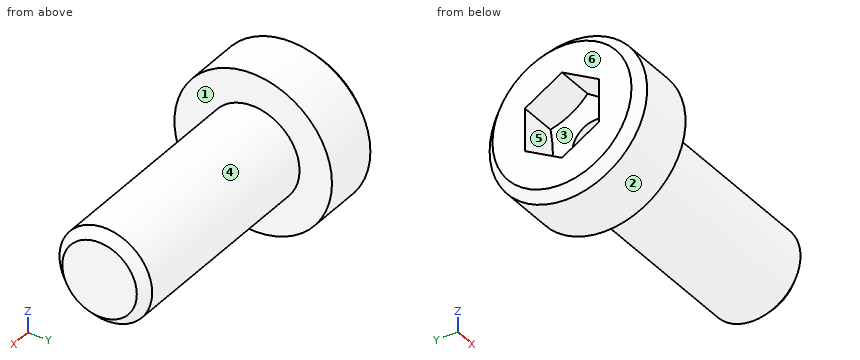
Autodesk Inventor part; units mm, degrees
ref_plane "Work Plane1" through (6, 0, 0) normal (0, 0.5, 0.8660254) x (1, 0, 0)
ref_plane "YZ Plane" through (0, 0, 0) normal (1, 0, 0) x (0, 1, 0)
ref_plane "XZ Plane" through (0, 0, 0) normal (0, 1, 0) x (-1, 0, 0)
sketch "Sketch1" plane through (0, 0, 0) normal (0, 0, 1) x (1, 0, 0)
  line L0 (1.2217, 0) -> (12, 0)
  line L1 (12, 0) -> (12, 2.5)
  line L2 (12, 2.5) -> (0, 2.5)
  line L3 (0, 2.5) -> (0, 4.25)
  line L4 (0, 4.25) -> (-3.5, 4.25)
  line L5 (-3.5, 4.25) -> (-3.5, 2.3094)
  line L6 (-3.5, 2.3094) -> (-1.5, 2.3094)
  line L7 (-1.5, 2.3094) -> (-0.8884, 1.25)
  line L8 (-6.6, 0) -> (15.1, 0)
  line L9 (0, -0.85) -> (0, 5.1)
  line L10 (-0.8884, 1.25) -> (0.5, 1.25)
  line L11 (0.5, 1.25) -> (1.2217, 0)
  line L12 (-3.5, 2.3094) -> (-3.5, 0) construction
  line L13 (-3.5, 3.75) -> (-3, 4.25)
  dimension "d0" = 3.5
  dimension "d1" = 2
  dimension "d2" = 60
  dimension "d3" = 5
  dimension "d4" = 4.6188
  dimension "d5" = 8.5
  dimension "d15" = 4
  dimension "d16" = 2.5
  dimension "d17" = 12
  dimension "d32" = 45
  dimension "d33" = 0.5
revolve "Body" add sketch "Sketch1" angle 360 about axis through (1.2217, 0, 0) along (1, 0, 0) contours L11 L10 L9 L2 L1 L0 | L10 L7 L6 L5 L13 L4 L3 L9 | L13 L5 L4
revolve "Chamfer2" cut sketch "Sketch1" angle 360 about axis through (-10, 0, 0) along (1, 0, 0) contours L13 L5 L4
sketch "Sketch2" plane through (-3.5, 0, 0) normal (-1, 0, 0) x (0, 0, 1)
  circle A0 centre (0, 0) radius 2.3094
  line L0 (0, -5.95) -> (0, 5.95)
  line L1 (-5.95, 0) -> (5.95, 0)
  line L2 (2.3094, 0) -> (1.1547, -2)
  line L3 (1.1547, -2) -> (-1.1547, -2)
  line L4 (-1.1547, -2) -> (-2.3094, 0)
  line L5 (-2.3094, 0) -> (-1.1547, 2)
  line L6 (-1.1547, 2) -> (1.1547, 2)
  line L7 (1.1547, 2) -> (2.3094, 0)
extrude "Slot" add sketch "Sketch2" against normal up to next contours L7 A0 | A0 L2 | L6 L0 A0 | A0 L0 L3 | L0 L6 A0 | A0 L3 L0 | L4 A0 | A0 L5
thread "Thread"
chamfer "Chamfer1" distance 0.4908 distance2 0.4908 1 edges at (12, -2.5, 0) measured on face at (12, -0.7741, -0.6858)
ref_plane "Work Plane1" through (6, 0, 0) normal (0, 0.5, 0.8660254) x (1, 0, 0)
equation "\"d0\" = KOH"
equation "\"d1\" = INTI"
equation "\"d3\" = GD"
equation "\"d4\" = 1.1547 * SW"
equation "\"d5\" = KOD"
equation "\"d15\" = INFT"
equation "\"d16\" = SDT"
equation "\"d17\" = NLG"
equation "\"d33\" = Cham"
equation "\"d7\" = GEL"
equation "\"d9\" = -0.5 * SPD + 0.5 * GD"
equation "\"d12\" = GUL"
equation "\"GD\" = NND"
equation "\"NLG\" = 12"
equation "\"GEL\" = 7.8"
equation "\"KOD\" = 8.5"
equation "\"KOH\" = 3.5"
equation "\"GUL\" = 0.61345 * PTC"
equation "\"SW\" = 4"
equation "\"INTI\" = 2"
equation "\"SPD\" = NND - 1.2269 * PTC"
equation "\"SDT\" = 2.5"
equation "\"INFT\" = 4"
equation "\"Cham\" = 0.5"
equation "\"TOA\" = 30deg"
equation "\"GD1\" = THREADDIA - 1.2269 * PTC"
equation "\"THREADDIA\" = 5"
equation "\"BDM\" = NND"
equation "\"FAWI\" = 45deg"
equation "\"RR\" = 0.1 * NND"
equation "\"PTC\" = 0.8"
equation "\"NND\" = 5"
equation "\"FAWI1\" = 45deg"
equation "\"GAL\" = 0.61345 * PTC"
equation "\"E0\" = 1.155 * SW"
properties part number "DIN 6912 - M5 x 12" material "Steel, Mild"
Geometry: final body of the model. Coordinates: model frame, mm. Face numbers are marked on the shaded views. A direction names the side the tool comes from. Give positions to 0.01 mm unless a question says otherwise; leave off trailing zeros. Write each loop counter-clockwise with the first axis right and the second up, starting at its lowest first coordinate (ties: lowest second). Pieces come first, ordered by that corner, then holes. Notation, with made-up numbers: (27, 86) - (53, 86) arc R23 cw to (53, 103) - close; hole circle Ø8 at (54.25, 30.5). An arc over 180 degrees is marked (long way). Return JSON: item names as keys, results as strings. Group by question number.
1) Mould query, pull axis Z, two halves, no side actions, for the marked faces 1, 2 and 3. Classes: released by +Z, released by -Z, zero draft, split by the parting line, or undercut.
2) Set-up query: the marked faces 4, 5 and 6. Return all of +Z, -Z, +X, -X, +Y, -Y with unobstructed straight access to the full face (end or side cutting, diameter ignored); none if empty.
3) Line query: line 1 (Z direction, x = 0.15, y = 0); line 2 (Z direction, x = -0.55, y = 0); line 3 (X direction, y = -2.5, z = 1.5). Output: solid intervals per line, ascending.
4) Section B-B on x = 6.25. Return the cut outline in (y, z).
5) First-contact query: P1, Ø1.5, axis at y = 2, z = 1.5, coming from the +X side; P2, Ø1, axis at x = 4, z = 0, coming from the -Y side; P3, Ø1.5, axis at y = 0, z = 0, coming from the -X side. Flat tips, straight axial feed; report the tip coordinate or a pass-through.
6) Section A-A on x = 0.25. Return the cut outline in (y, z), plus the area to 3 significant figures.
Filled in:
{
 "1": {"face 1": "zero draft", "face 2": "split by the parting line", "face 3": "undercut"},
 "2": {"face 4": "+X", "face 5": "-X", "face 6": "+Z, -Z, -X, +Y, -Y"},
 "3": {"line 1": "z = -2.5 to -1.25, 1.25 to 2.5", "line 2": "z = -4.25 to -1.25, 1.25 to 4.25", "line 3": "x = -3.5 to 0"},
 "4": {"outline": "circle Ø5 at (0, 0)"},
 "5": {"P1": "stops at x = 12", "P2": "stops at y = -2.5", "P3": "stops at x = 0.79"},
 "6": {"outline": "circle Ø5 at (0, 0); hole circle Ø2.5 at (0, 0)", "area": "14.7 mm^2"}
}
